Model file for the job. Use its own axes, mm. A direction names the side the tool comes from. Coordinates: 2 decimals unless noted, no trailing zeros. Write each loop counter-clockwise with the first axis right and the second up, starting at its lowest first coordinate (ties: lowest second). Pieces come first, ordered by that corner, then holes. Notation, with made-up numbers: (-39, 61.25) -> (4, 61.25) arc R12 ccw to (4, 69.25) -> close; hole circle Ø6 at (47, -6.75). An arc over 180 degrees is marked (long way). Answer as a JSON object with one key per item and string values. Group by question number.
from build123d import *

# Parameters (mm, degrees)
SKETCH1_W           = 55
SKETCH1_H           = 20
SKETCH1_R           = 2.15
BOSS_EXTRUDE1_DEPTH = 5
SKETCH2_W           = 55
SKETCH2_H           = 3
BOSS_EXTRUDE2_DEPTH = 75
CUT_EXTRUDE1_DEPTH  = 75


with BuildPart() as part:
    # Sketch1 → Boss-Extrude1 (new body)
    with BuildSketch(Plane(origin=(0, 0, 0), x_dir=(1, 0, 0), z_dir=(0, 1, 0))):
        Rectangle(SKETCH1_W, SKETCH1_H)
        with Locations((-20, 0)):
            Circle(SKETCH1_R, mode=Mode.SUBTRACT)
        with Locations((20, 0)):
            Circle(SKETCH1_R, mode=Mode.SUBTRACT)
    extrude(amount=BOSS_EXTRUDE1_DEPTH)

    # Sketch2 → Boss-Extrude2 (add)
    with BuildSketch(Plane(origin=(0, 5, 0), x_dir=(1, 0, 0), z_dir=(0, 1, 0))):
        with Locations((0, -8.5)):
            Rectangle(SKETCH2_W, SKETCH2_H)
    extrude(amount=BOSS_EXTRUDE2_DEPTH)

    # Sketch3 → Cut-Extrude1 (cut)
    with BuildSketch(Plane(origin=(0, 0, 7), x_dir=(-1, 0, 0), z_dir=(0, 0, -1))):
        with BuildLine():
            Line((-20.85, 69.022285576), (-20.85, 20.608862032))
            ThreePointArc((-20.85, 20.608862032), (-22.5, 18.958862032), (-24.15, 20.608862032))
            Line((-24.15, 20.608862032), (-24.15, 69.022285576))
            ThreePointArc((-24.15, 69.022285576), (-22.5, 70.672285576), (-20.85, 69.022285576))
        make_face()
        with BuildLine():
            Line((20.85, 69.022285576), (20.85, 20.608862032))
            ThreePointArc((20.85, 20.608862032), (22.5, 18.958862032), (24.15, 20.608862032))
            Line((24.15, 20.608862032), (24.15, 69.022285576))
            ThreePointArc((24.15, 69.022285576), (22.5, 70.672285576), (20.85, 69.022285576))
        make_face()
    extrude(amount=-CUT_EXTRUDE1_DEPTH, mode=Mode.SUBTRACT)


solid = part.part
(1) Pin check, flat tips, straight feed: pin 1 (16.5 mm diameter, centred on x = 5.5, y = 36.5, fed in from -Z); pin 2 (3 mm diameter, centred on x = 12.5, z = -4.5, fed in from +Y). Stop position of each tip, or through.
(2) 3-axis set-ups, long thin cutter, end or side, ignore diameter. For faces 1 (the face through (20.85, 45, 8)), 2 (the face through (0, 5, -2)), 3 (the face through (0, 80, 8)): which of +Z, -Z, +X, -X, +Y, -Y reach the whole face in a straight line?
(3) Cut at B-B on y = 49.5. List the corners of the cut face in (x, z), plus the area to 3 significant figures.
(4) Cut at C-C on x = -20. List the corners of the cut face in (y, z), plus the area to 4 significant figures.
(5) Cut at A-A on z = 0. List the corners of the cut face in (x, y).
(6) Pull direction Z, two halves, no side cores. Call faces 4 (the face through (27.5, 30.9, 7.5)), 5 (the face through (-22.15, 2.46, -0.09)), 6 (the face through (0, 42, 7)), 7 (the face through (17.85, 2.46, -0.09)): released by +Z, released by -Z, zero draft, split by the parting line, or undercut.
(7) Cut at D-D on z = 8.5. List the corners of the cut face in (x, y).
(8) Wall check: probe 1 along X at (y, z) = (1.1, 0); probe 2 along X at (y, z) = (58.5, 9); probe 3 along Z at (x, y) = (20, 2). Give the ranges that are in metal, low to high.
Results found:
{
 "1": {"pin 1": "stops at z = 7", "pin 2": "stops at y = 5"},
 "2": {"face 1": "+Z, -Z", "face 2": "-Z, +X, -X, +Y", "face 3": "+Z, -Z, +X, -X, +Y"},
 "3": {"outline": "(-27.5, 7) -> (-24.15, 7) -> (-24.15, 10) -> (-27.5, 10) -> close; (-20.85, 7) -> (20.85, 7) -> (20.85, 10) -> (-20.85, 10) -> close; (24.15, 7) -> (27.5, 7) -> (27.5, 10) -> (24.15, 10) -> close", "area": "145 mm²"},
 "4": {"outline": "(0, -10) -> (5, -10) -> (5, -2.15) -> (0, -2.15) -> close; (0, 2.15) -> (5, 2.15) -> (5, 7) -> (80, 7) -> (80, 10) -> (0, 10) -> close", "area": "303.5 mm²"},
 "5": {"outline": "(-27.5, 0) -> (-22.15, 0) -> (-22.15, 5) -> (-27.5, 5) -> close; (-17.85, 0) -> (17.85, 0) -> (17.85, 5) -> (-17.85, 5) -> close; (22.15, 0) -> (27.5, 0) -> (27.5, 5) -> (22.15, 5) -> close"},
 "6": {"face 4": "zero draft", "face 5": "undercut", "face 6": "released by -Z", "face 7": "undercut"},
 "7": {"outline": "(-27.5, 0) -> (27.5, 0) -> (27.5, 80) -> (-27.5, 80) -> close; hole (-24.15, 20.61) arc R1.65 ccw to (-20.85, 20.61) -> (-20.85, 69.02) arc R1.65 ccw to (-24.15, 69.02) -> close; hole (20.85, 20.61) arc R1.65 ccw to (24.15, 20.61) -> (24.15, 69.02) arc R1.65 ccw to (20.85, 69.02) -> close"},
 "8": {"probe 1": "x = -27.5 to -22.15, -17.85 to 17.85, 22.15 to 27.5", "probe 2": "x = -27.5 to -24.15, -20.85 to 20.85, 24.15 to 27.5", "probe 3": "z = -10 to -2.15, 2.15 to 10"}
}
